Here's how the part is built. I have some questions about the finished solid (model axes, mm). A direction names the side the tool comes from. Round coordinates to 2 decimals unless told otherwise and drop trailing zeros. Order: outer loops, then holes, each group sorted by start corner. A loop starts at its lowest first (then second) coordinate and runs counter-clockwise, first axis right, second up.
```python
from build123d import *

# Parameters (mm, degrees)
F0_W     = 31
F0_H     = 8.8
F0_H_2   = 22.2
F0_R     = 2.6
F1_DEPTH = 4
F2_DEPTH = 4.4
F3_W     = 31
F3_H     = 4.4
F5_R     = 2
F6_DEPTH = 31.001
F7_R     = 2


with BuildPart() as f1:
    # F0 (on Top) → F1 (new body)
    with BuildSketch(Plane.XY):
        with Locations((-56.2723039389, 48.8844518721)):
            Rectangle(F0_W, F0_H)
        with Locations((-56.2723039389, 33.3844518721)):
            Rectangle(F0_W, F0_H_2)
        with Locations((-56.2723039389, 33.3844518721)):
            Circle(F0_R, mode=Mode.SUBTRACT)
    extrude(amount=-F1_DEPTH)

    # F0 (on Top) → F2 (join)
    with BuildSketch(Plane.XY):
        with Locations((-56.2723039389, 48.8844518721)):
            Rectangle(F0_W, F0_H)
    extrude(amount=F2_DEPTH)

    # F3 (on face) → F4 (revolve)
    with BuildSketch(Plane.XY.offset(4.4)):
        with Locations((-56.2723039389, 46.6844518721)):
            Rectangle(F3_W, F3_H)
    revolve(axis=Axis((-56.2723039389, 48.8844518721, 4.4), (-1, 0, 0)))

    # F5 (on face) → F6 (cut, through all)
    with BuildSketch(Plane.YZ.offset(-40.7723039389)):
        with Locations((48.8844518721, 4.4)):
            Circle(F5_R)
    extrude(amount=-F6_DEPTH, mode=Mode.SUBTRACT)

    # F7
    f7_edges = [f1.edges().sort_by_distance(p)[0] for p in [
        (-56.272304, 44.484452, 0),
        (-40.772304, 22.284452, -2),
        (-71.772304, 22.284452, -2),
        (-56.272304, 22.284452, 0),
        (-40.772304, 33.384452, 0),
        (-71.772304, 33.384452, 0),
        (-71.772304, 53.284452, 0.2),
        (-40.772304, 53.284452, 0.2),
        (-71.772304, 48.884452, 8.8),
        (-40.772304, 48.884452, 8.8),
    ]]
    fillet(f7_edges, radius=F7_R)


solid = f1.part
```
1) We'd pull the mould along X, two halves only. Please class faces 5 (the flat face through (-40.772, 41.8, -2.2)), 6 (the cylindrical face through (-53.87, 32.39, -1.97)), 7 (the cylindrical face through (-71.202, 22.886, -3.014)): +X half, -X half, draft (parallel to the pull), parting line (faces both ways), or undercut.
2) If we section it at C-C (z = -2.5): Write out the boundary of the cut face in (x, y).
3) If we section it at A-A (x = -64.5): Write out the boundary of the cut face in (y, z), plus the area to 3 significant figures.
4) For faces 1 (the cylindrical face through (-41.374, 33.512, -0.57)), 2 (the cylindrical face through (-71.202, 45.086, 3.217)), 3 (the flat face through (-71.772, 41.8, -2.2)), 4 (the flat face through (-56, 44.484, 3)), which set-ups out of +Z, -Z, +X, -X, +Y, -Y let a thin tool reach every point of the face, with its end or its side?
5) I'm going to push flat-ended pins straight in: pin 1 (2 mm diameter, centred on y = 38.5, z = -0.5, fed in from +X); pin 2 (8.5 mm diameter, centred on x = -56.27, y = 33.38, fed in from +Z); pin 3 (3 mm diameter, centred on x = -67, z = 6, fed in from -Y). Where does each tip first touch, or does it pass through?
6) I need wall thicknesses on line 1 (Z direction, x = -50, y = 29); line 2 (Y direction, x = -52, z = 3.25); line 3 (Z direction, x = -64.5, y = 50). Which ranges of each line are inside material? Lowest first, please.
7) If we section it at B-B (y = 40.5): Write out the boundary of the cut face in (x, z).
Solutions:
1. face 5: +X half
1. face 6: undercut
1. face 7: -X half
2. outline: (-71.77, 24.28) arc R2 ccw to (-69.77, 22.28) - (-42.77, 22.28) arc R2 ccw to (-40.77, 24.28) - (-40.77, 51.28) arc R2 ccw to (-42.77, 53.28) - (-69.77, 53.28) arc R2 ccw to (-71.77, 51.28) - close; hole circle Ø5.2 at (-56.27, 33.38)
3. outline: (22.28, -4) - (53.28, -4) - (53.28, 4.4) arc R4.4 ccw to (44.48, 4.4) - (44.48, 2) arc R2 cw to (42.48, 0) - (24.28, 0) arc R2 ccw to (22.28, -2) - close; hole circle Ø4 at (48.88, 4.4)
3. area: 181 mm2
4. face 1: +Z, +X, -Y
4. face 2: +Z, -X, -Y
4. face 3: +Z, -Z, -X, +Y, -Y
4. face 4: +Z, +X, -X, -Y
5. pin 1: stops at x = -40.84
5. pin 2: stops at z = 0
5. pin 3: stops at y = 44.49
6. line 1: z = -4 to 0
6. line 2: y = 44.48 to 47.25, 50.52 to 53.28
6. line 3: z = -4 to 2.74, 6.06 to 8.66
7. outline: (-71.77, -4) - (-40.77, -4) - (-40.77, -2) arc R2 ccw to (-42.77, 0) - (-69.77, 0) arc R2 ccw to (-71.77, -2) - close
